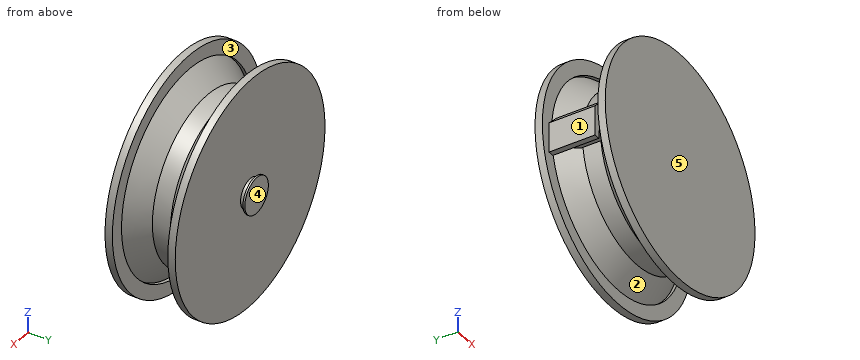
Autodesk Inventor part; units mm, degrees
ref_plane "YZ Plane" through (0, 0, 0) normal (1, 0, 0) x (0, 1, 0)
ref_plane "XZ Plane" through (0, 0, 0) normal (0, 1, 0) x (-1, 0, 0)
ref_plane "XY Plane" through (0, 0, 0) normal (0, 0, 1) x (1, 0, 0)
sketch "Sketch1" plane through (0, 0, 0) normal (0, 0, 1) x (1, 0, 0)
  line L0 (0, 0) -> (27.5, 0)
  line L1 (27.5, 17) -> (0, 17)
  line L2 (0, 17) -> (0, 0)
  line L3 (0, 8.5) -> (32.996, 8.5) construction
  line L4 (27.5, 17) -> (20.3677, 8.5)
  line L5 (27.5, 17) -> (38.596, 17) construction
  line L6 (27.5, 0) -> (20.3677, 8.5)
  dimension "d0" = 27.5
  dimension "d2" = 17
  dimension "d3" = 27.5
  dimension "d4" = 130
revolve "Revolution1" add sketch "Sketch1" angle 360 about axis through (0, 17, 0) along (0, -1, 0)
sketch "Sketch4" plane through (0, 0, 0) normal (0, -1, 0) x (1, 0, 0)
  circle A0 centre (0, 0) radius 27.5
  circle A1 centre (0, 0) radius 31.31
  dimension "d12" = 3.81
extrude "Extrusion2" add sketch "Sketch4" along normal blind 1 and the other way blind 1
ref_plane "Work Plane1" through (0, 8.5, 0) normal (0, -1, 0) x (1, 0, 0)
sketch "Sketch5" plane through (0, 0, 0) normal (0, -1, 0) x (1, 0, 0)
  circle A0 centre (0, 0) radius 27.5
extrude "Extrusion3" add sketch "Sketch5" along normal blind 1
mirror "Mirror1" about plane through (0, 8.5, 0) normal (0, -1, 0) of "Extrusion2"
sketch "Sketch6" plane through (0, 17, 0) normal (0, 1, 0) x (1, 0, 0)
  circle A0 centre (0, 0) radius 27.5
extrude "Extrusion4" add sketch "Sketch6" along normal blind 1
chamfer "Chamfer1" distance 3.175 angle 45 1 edges at (-20.3677, 8.5, 0)
sketch "Sketch7" plane through (0, 18, 0) normal (0, 1, 0) x (1, 0, 0)
  circle A0 centre (0, 0) radius 31.31 construction
  line L0 (0, 31.31) -> (0, -31.31) construction
  circle A1 centre (0, 0) radius 22.4085
  circle A2 centre (0, 0) radius 27.5
  circle A3 centre (0, 0) radius 22.4085
  circle A4 centre (0, 0) radius 27.5 construction
  line L1 (-27.5, 14.9688) -> (-27.5, 0) construction
  circle A5 centre (0, 0) radius 27.5 construction
  line L2 (-27.5, -14.9688) -> (-27.5, 0) construction
ref_plane "Work Plane2" through (-27.5, 18, 14.9688) normal (-1, 0, 0) x (0, 0, -1)
sketch "Sketch8" plane through (-27.5, 18, 14.9688) normal (-1, 0, 0) x (0, 0, -1)
  line L0 (37.3773, 7.0678) -> (37.3773, 11.9322) construction
  line L1 (37.3773, 9.5) -> (-7.4397, 9.5) construction
  line L2 (-7.4397, 7.0678) -> (-7.4397, 11.9322) construction
  line L3 (18.361, 15.7245) -> (11.5766, 15.7245)
  line L4 (11.5766, 15.7245) -> (11.5766, 3.2755)
  line L5 (11.5766, 3.2755) -> (18.361, 3.2755)
  line L6 (18.361, 3.2755) -> (18.361, 15.7245)
  line L7 (18.361, 15.7245) -> (11.5766, 3.2755) construction
  line L8 (11.5766, 15.7245) -> (18.361, 3.2755) construction
  point P0 (14.9688, 18)
  point P1 (14.9688, 9.5)
extrude "Extrusion5" add sketch "Sketch8" along normal blind 3 and the other way blind 5
chamfer "Chamfer2" distance 3.175 angle 45 1 edges at (-30.5, 8.5, 3.3922)
sketch "Sketch9" plane through (-25.3648, 2.2755, -3.3922) normal (0, 0, -1) x (-1, 0, 0)
  line L0 (5.1352, 0) -> (1.9602, 0)
  line L1 (0, 12.449) -> (5.1352, 12.449)
  line L2 (3.5477, 0) -> (5.1352, 0)
  line L3 (5.1352, 0) -> (5.1352, 12.449)
  line L4 (5.1352, 12.449) -> (3.5477, 12.449)
  line L5 (3.5477, 12.449) -> (3.5477, 0)
  point P0 (-25.3648, -2.2755)
extrude "Extrusion6" add sketch "Sketch9" along normal blind 4.5
fillet "Fillet2" radius 3.175 1 edges at (-28.9125, 8.5, -3.3922)
sketch "Sketch10" plane through (0, 18, 0) normal (0, 1, 0) x (1, 0, 0)
  circle A0 centre (0, 0) radius 4
  dimension "d35" = 8
extrude "Extrusion7" add sketch "Sketch10" along normal blind 1.5
sketch "Sketch11" plane through (0, 19.5, 0) normal (0, 1, 0) x (1, 0, 0)
  circle A0 centre (0, 0) radius 4.9245
  dimension "d38" = 9.849
extrude "Extrusion8" add sketch "Sketch11" along normal mid plane 0.5
properties part number "WireRewindDRUM"
Build history of the part. All positions in model axes, mm. Face numbers are marked on the shaded views. A direction names the side the tool comes from. Round coordinates to 2 decimals unless told otherwise and drop trailing zeros. Use CSV: the item, a comma, the result in double quotes.
(1) Wall check: line 1 (Z direction, x = 0, y = 0.7); line 2 (Z direction, x = 0, y = 0.8); line 3 (Y direction, x = 15, z = -25). Give the ranges that are in metal, low to high.
Response:
line 1,"-31.31 to -27.5, -26.91 to 26.91, 27.5 to 31.31"
line 2,"-31.31 to -27.5, -26.83 to 26.83, 27.5 to 31.31"
line 3,"-1 to 1, 16 to 18"
(2) 3-axis set-ups, long thin cutter, end or side, ignore diameter. For the marked faces 1 and 2: which of +Z, -Z, +X, -X, +Y, -Y reach the whole face in a straight line?
Response:
face 1,"+Z, -Z, -X"
face 2,"none"
(3) Mould opens along Y. For the marked faces 3, 4 and 5 say: pulls with the +Y half, pulls with the -Y half, needs draft (parallel to the pull), parting line crosses it, or undercut.
Response:
face 3,"undercut"
face 4,"pulls with the +Y half"
face 5,"pulls with the -Y half"
(4) Pin check, flat tips, straight feed: P1, Ø0.7, axis at y = 7, z = -7, coming from the +X side; P2, Ø5, axis at x = 24, z = 24, coming from the -Y side; P3, Ø2, axis at x = -4, z = 12, coming from the +Y side; P4, Ø6.5, axis at y = 8, z = -4.5, coming from the -X side. Stop position of each tip, or through.
Response:
P1,"x = 21.4"
P2,"through"
P3,"y = 18"
P4,"x = -30.5"
